Check sheet for the modelled part. Datum: model origin and axes. Units: mm. A direction names the side the tool comes from. Round coordinates to 2 decimals unless told otherwise and drop trailing zeros. Write each loop counter-clockwise with the first axis right and the second up, starting at its lowest first coordinate (ties: lowest second). Pieces come first, ordered by that corner, then holes.
from build123d import *

# Parameters (mm, degrees)
SKETCH1_W                = 51
SKETCH1_H                = 53.5
BOSS_EXTRUDE1_DEPTH      = 54.25
SKETCH2_W                = 43
SKETCH2_H                = 43
CUT_EXTRUDE1_DEPTH       = 50.75
SKETCH3_W                = 43
SKETCH3_H                = 3.5
CUT_EXTRUDE2_DEPTH       = 37.5
CUT_EXTRUDE3_DEPTH       = 76
SKETCH5_R                = 9.673114497
SKETCH5_R_2              = 5.390775308
SKETCH5_R_3              = 5.456912487
CUT_EXTRUDE4_DEPTH       = 76
SKETCH6_R                = 14
SKETCH6_R_2              = 1.75
CUT_EXTRUDE5_DEPTH       = 76
SKETCH7_R                = 5
CUT_EXTRUDE6_DEPTH       = 76
CUT_EXTRUDE7_DEPTH       = 27
FILLET2_R                = 1
SKETCH12_R               = 1.75
CUT_EXTRUDE8_DEPTH       = 15
BOSS_EXTRUDE4_DEPTH      = 10
BOSS_EXTRUDE4_DEPTH_BACK = 61
SKETCH13_W               = 16.75
SKETCH13_H               = 3.5
SKETCH14_W               = 71
SKETCH14_H               = 1.75
BOSS_EXTRUDE5_DEPTH      = 15
SKETCH15_R               = 1.75
CUT_EXTRUDE9_DEPTH       = 10
SKETCH16_R               = 1.75
CUT_EXTRUDE10_DEPTH      = 10
CUT_EXTRUDE11_REACH      = 95.245
FILLET3_R                = 5
FILLET4_R                = 1
CUT_EXTRUDE12_DEPTH      = 2.5


with BuildPart() as part:
    # Sketch1 → Boss-Extrude1 (new body)
    with BuildSketch(Plane.XY):
        with Locations((-26.432354029, 2.021717979)):
            Rectangle(SKETCH1_W, SKETCH1_H)
    extrude(amount=BOSS_EXTRUDE1_DEPTH)

    # Sketch2 → Cut-Extrude1 (cut)
    with BuildSketch(Plane.XY.offset(54.25)):
        with Locations((-26.432354029, 3.771717979)):
            Rectangle(SKETCH2_W, SKETCH2_H)
    extrude(amount=-CUT_EXTRUDE1_DEPTH, mode=Mode.SUBTRACT)

    # Sketch3 → Cut-Extrude2 (cut)
    with BuildSketch(Plane.XY.offset(54.25)):
        with Locations((-26.432354029, 27.021717979)):
            Rectangle(SKETCH3_W, SKETCH3_H)
    extrude(amount=-CUT_EXTRUDE2_DEPTH, mode=Mode.SUBTRACT)

    # Sketch4 → Cut-Extrude3 (cut)
    with BuildSketch(Plane.ZY.offset(51.932354029)):
        with BuildLine():
            Line((16.75, 28.771717979), (54.25, 28.771717979))
            Line((54.25, 28.771717979), (54.25, -7.074674815))
            ThreePointArc((54.25, -7.074674815), (27.422353926, 2.398250742), (16.75, 28.771717979))
        make_face()
    extrude(amount=-CUT_EXTRUDE3_DEPTH, mode=Mode.SUBTRACT)

    # Sketch5 → Cut-Extrude4 (cut)
    with BuildSketch(Plane.ZY.offset(51.932354029)):
        with Locations(Location((14.525222974, -6.808047023, 0), (0, 0, 270))):
            Circle(SKETCH5_R)
        with Locations(Location((34.168969833, -12.297713654, 0), (0, 0, 270))):
            Circle(SKETCH5_R_2)
        with Locations(Location((9.035556344, 13.166402645, 0), (0, 0, 270))):
            Circle(SKETCH5_R_3)
    extrude(amount=-CUT_EXTRUDE4_DEPTH, mode=Mode.SUBTRACT)

    # Sketch6 → Cut-Extrude5 (cut)
    with BuildSketch(Plane.XY.offset(3.5)):
        with Locations((-26.432354029, 3.771717979)):
            Circle(SKETCH6_R)
        with Locations((-10.932354029, 19.271717979)):
            Circle(SKETCH6_R_2)
        with Locations((-41.932354029, 19.271717979)):
            Circle(SKETCH6_R_2)
        with Locations((-41.932354029, -11.728282021)):
            Circle(SKETCH6_R_2)
        with Locations((-10.932354029, -11.728282021)):
            Circle(SKETCH6_R_2)
    extrude(amount=-CUT_EXTRUDE5_DEPTH, mode=Mode.SUBTRACT)

    # Sketch7 → Cut-Extrude6 (cut)
    with BuildSketch(Plane(origin=(0, 0, 0), x_dir=(-1, 0, 0), z_dir=(0, 0, -1))):
        with Locations((26.432354029, -24.728282021)):
            Circle(SKETCH7_R)
    extrude(amount=-CUT_EXTRUDE6_DEPTH, mode=Mode.SUBTRACT)

    # Sketch8 → Cut-Extrude7 (cut)
    with BuildSketch(Plane.XZ.offset(24.728282021)):
        Polygon((-26.432354029, 46.625), (-6.932354029, 27.125), (-26.432354029, 7.625), (-45.932354029, 27.125), align=None)
        Polygon((-13.361286217, 40.625), (-4.932354029, 40.625), (-4.932354029, 32.196067812), align=None)
        Polygon((-4.932354029, 13.625), (-13.361286217, 13.625), (-4.932354029, 22.053932188), align=None)
        Polygon((-47.932354029, 13.625), (-39.503421841, 13.625), (-47.932354029, 22.053932188), align=None)
        Polygon((-47.932354029, 40.625), (-39.007101497, 40.625), (-47.932354029, 31.699747468), align=None)
    extrude(amount=-CUT_EXTRUDE7_DEPTH, mode=Mode.SUBTRACT)

    # Fillet2
    fillet2_edges = [part.edges().sort_by_distance(p)[0] for p in [
        (-47.932354029, -21.228282021, 31.699747468),
        (-4.932354029, -21.228282021, 32.196067812),
        (-4.932354029, -21.228282021, 22.053932188),
        (-47.932354029, -21.228282021, 22.053932188),
        (-13.361286217, -21.228282021, 13.625),
        (-39.503421841, -21.228282021, 13.625),
        (-26.432354029, -18.728282021, 7.625),
        (-4.932354029, -21.228282021, 13.625),
        (-47.932354029, -21.228282021, 13.625),
        (-45.932354029, -21.228282021, 27.125),
        (-6.932354029, -21.228282021, 27.125),
        (-4.932354029, -21.228282021, 40.625),
        (-47.932354029, -21.228282021, 40.625),
        (-39.007101497, -21.228282021, 40.625),
        (-13.361286217, -21.228282021, 40.625),
        (-26.432354029, -18.728282021, 46.625),
    ]]
    fillet(fillet2_edges, radius=FILLET2_R)

    # Sketch12 → Cut-Extrude8 (cut)
    with BuildSketch(Plane.XZ.offset(24.728282021)):
        with Locations(Location((-11.432354029, 46.25, 0), (0, 0, 270))):
            Circle(SKETCH12_R)
        with Locations(Location((-41.432354029, 46.25, 0), (0, 0, 270))):
            Circle(SKETCH12_R)
        with Locations(Location((-11.432354029, 8, 0), (0, 0, 270))):
            Circle(SKETCH12_R)
        with Locations(Location((-41.432354029, 8, 0), (0, 0, 270))):
            Circle(SKETCH12_R)
    extrude(amount=-CUT_EXTRUDE8_DEPTH, mode=Mode.SUBTRACT)

    # Sketch13 → Boss-Extrude4 (add, two sides: drawn at the far end of the back side and taken through both)
    with BuildSketch(Plane.ZY.offset(51.932354029).offset(-BOSS_EXTRUDE4_DEPTH_BACK)):
        with Locations((8.375, 27.021717979)):
            Rectangle(SKETCH13_W, SKETCH13_H)
    extrude(amount=BOSS_EXTRUDE4_DEPTH + BOSS_EXTRUDE4_DEPTH_BACK)

    # Sketch14 → Boss-Extrude5 (add)
    with BuildSketch(Plane(origin=(0, 28.771717979, 0), x_dir=(1, 0, 0), z_dir=(0, 1, 0))):
        with Locations((-26.432354029, -0.875)):
            Rectangle(SKETCH14_W, SKETCH14_H)
    extrude(amount=BOSS_EXTRUDE5_DEPTH)

    # Sketch15 → Cut-Extrude9 (cut)
    with BuildSketch(Plane.XZ.offset(-25.271717979)):
        with Locations((-56.932354029, 9.25)):
            Circle(SKETCH15_R)
        with Locations((4.067645971, 9.25)):
            Circle(SKETCH15_R)
    extrude(amount=-CUT_EXTRUDE9_DEPTH, mode=Mode.SUBTRACT)

    # Sketch16 → Cut-Extrude10 (cut)
    with BuildSketch(Plane(origin=(0, 0, 0), x_dir=(-1, 0, 0), z_dir=(0, 0, -1))):
        with Locations((54.432354029, 36.271717979)):
            Circle(SKETCH16_R)
        with Locations((-1.567645971, 36.271717979)):
            Circle(SKETCH16_R)
        with Locations((44.432354029, 36.271717979)):
            Circle(SKETCH16_R)
        with Locations((8.432354029, 36.271717979)):
            Circle(SKETCH16_R)
    extrude(amount=-CUT_EXTRUDE10_DEPTH, mode=Mode.SUBTRACT)

    # Cut-Extrude11: up to this face of the body (flat: up to its plane)
    cut_extrude11_end = Plane(part.part.faces().sort_by_distance((-26.432354029, -17.120170189, 3.5))[0])
    # Sketch17 → Cut-Extrude11 (cut, up to the picked face)
    with BuildSketch(Plane.XY.offset(54.25), mode=Mode.PRIVATE) as cut_extrude11_sk1:
        with BuildLine():
            Line((-17.488082119, -19.228282021), (-4.932354029, -19.228282021))
            Line((-4.932354029, -19.228282021), (-4.932354029, -17.728282021))
            Line((-4.932354029, -17.728282021), (-18.606116108, -17.728282021))
            ThreePointArc((-18.606116108, -17.728282021), (-18.013624909, -18.453331822), (-17.488082119, -19.228282021))
        make_face()
    cut_extrude11_tool1 = split(extrude(cut_extrude11_sk1.sketch, amount=-CUT_EXTRUDE11_REACH, mode=Mode.PRIVATE), bisect_by=cut_extrude11_end, keep=Keep.BOTH, mode=Mode.PRIVATE)
    # Sketch17 → Cut-Extrude11 (cut, up to the picked face)
    with BuildSketch(Plane.XY.offset(54.25), mode=Mode.PRIVATE) as cut_extrude11_sk2:
        with BuildLine():
            Line((-35.376625939, -19.228282021), (-47.932354029, -19.228282021))
            Line((-47.932354029, -19.228282021), (-47.932354029, -17.728282021))
            Line((-47.932354029, -17.728282021), (-34.25859195, -17.728282021))
            ThreePointArc((-34.25859195, -17.728282021), (-34.851083149, -18.453331822), (-35.376625939, -19.228282021))
        make_face()
    cut_extrude11_tool2 = split(extrude(cut_extrude11_sk2.sketch, amount=-CUT_EXTRUDE11_REACH, mode=Mode.PRIVATE), bisect_by=cut_extrude11_end, keep=Keep.BOTH, mode=Mode.PRIVATE)
    add(cut_extrude11_tool1.solids().sort_by(Axis((-11.476334, -18.467624, 54.25), (0, 0, -1)))[0], mode=Mode.SUBTRACT)
    add(cut_extrude11_tool2.solids().sort_by(Axis((-41.388374, -18.467624, 54.25), (0, 0, -1)))[0], mode=Mode.SUBTRACT)

    # Fillet3
    fillet3_edges = [part.edges().sort_by_distance(p)[0] for p in [
        (-2.932354029, -7.074674815, 54.25),
        (-49.932354029, -7.074674815, 54.25),
    ]]
    fillet(fillet3_edges, radius=FILLET3_R)

    # Fillet4
    fillet4_edges = [part.edges().sort_by_distance(p)[0] for p in [
        (-51.932354029, 25.271717979, 8.375),
        (-0.932354029, 25.271717979, 8.375),
        (-0.932354029, -24.728282021, 27.125),
        (-51.932354029, -24.728282021, 27.125),
    ]]
    fillet(fillet4_edges, radius=FILLET4_R)

    # Sketch19 → Cut-Extrude12 (cut)
    with BuildSketch(Plane(origin=(0, -19.228282021, 0), x_dir=(1, 0, 0), z_dir=(0, 1, 0))):
        Polygon((-44.182354029, -9.58771324), (-41.432354029, -11.175426481), (-38.682354029, -9.58771324), (-38.682354029, -6.41228676), (-41.432354029, -4.824573519), (-44.182354029, -6.41228676), align=None)
        Polygon((-11.432354029, -4.824573519), (-14.182354029, -6.41228676), (-14.182354029, -9.58771324), (-11.432354029, -11.175426481), (-8.682354029, -9.58771324), (-8.682354029, -6.41228676), align=None)
        Polygon((-38.682354029, -47.83771324), (-38.682354029, -44.66228676), (-41.432354029, -43.074573519), (-44.182354029, -44.66228676), (-44.182354029, -47.83771324), (-41.432354029, -49.425426481), align=None)
        Polygon((-8.682354029, -47.83771324), (-8.682354029, -44.66228676), (-11.432354029, -43.074573519), (-14.182354029, -44.66228676), (-14.182354029, -47.83771324), (-11.432354029, -49.425426481), align=None)
    extrude(amount=-CUT_EXTRUDE12_DEPTH, mode=Mode.SUBTRACT)


solid = part.part
1. Release check for a two-part mould opening along Z. For faces 1 (the flat face through (-42.83, -20.46, 48.62)), 2 (the flat face through (6, 25.272, 8)), 3 (the flat face through (-36, -7, 3.5)), 4 (the flat face through (-8.682, -20, 8)) record: released by +Z, released by -Z, zero draft, split by the parting line, or undercut.
2. Sectioned sample at B-B, the plane y = 12.5. Enter the section's corners in (x, z).
3. Scan lines: line 1 along Z through (x, y) = (-1, 13.5); line 2 along X through (y, z) = (9, 5); line 3 along Y through (x, z) = (-44, 9.5). Record each from-to range of solid material in increasing order.
4. Go/stop test with flat-tipped pins: pin 1 (3 mm diameter, centred on x = -51.5, z = 28, fed in from -Y); pin 2 (3 mm diameter, centred on x = -41.43, z = 8, fed in from -Y); pin 3 (3 mm diameter, centred on x = -18.5, y = 18, fed in from +Z); pin 4 (6 mm diameter, centred on x = -10.5, z = 47, fed in from +Y). Record where each tip stops, or that it passes through.
5. Sectioned sample at D-D, the plane z = 32. Enter the section's corners in (x, y), plus the area to 3 significant figures.
6. Sectioned sample at C-C, the plane x = -20.5. Enter the section's corners in (y, z), plus the area to 3 significant figures.
7. Sectioned sample at A-A, the plane z = 23. Enter the section's corners in (x, y), plus the area to 3 significant figures.
8. Set-up check for faces 5 (the flat face through (-27, 25.272, 10)), 6 (the flat face through (-40.04, -20.46, 5.63)), 7 (the flat face through (-51.932, -5, 27)), 8 (the flat face through (-16.56, -21.28, 17.5)), 9 (the cylindrical face through (-40.504, -21.94, 40.023)): record each of +Z, -Z, +X, -X, +Y, -Y from which the full face is reachable in a straight line by a thin tool's end or side.
Computed values:
1. face 1: undercut
1. face 2: zero draft
1. face 3: released by +Z
1. face 4: undercut
2. outline: (-51.93, 0) - (-37.38, 0) - (-37.38, 3.5) - (-47.93, 3.5) - (-47.93, 3.62) - (-51.93, 3.62) - close; (-51.93, 14.45) - (-47.93, 14.45) - (-47.93, 20.11) - (-51.93, 20.11) - close; (-15.49, 0) - (-0.93, 0) - (-0.93, 3.62) - (-4.93, 3.62) - (-4.93, 3.5) - (-15.49, 3.5) - close; (-4.93, 14.45) - (-0.93, 14.45) - (-0.93, 20.11) - (-4.93, 20.11) - close
3. line 1: z = 0 to 3.59, 14.48 to 19.65
3. line 2: x = -51.93 to -47.93, -4.93 to -0.93
3. line 3: y = -24.73 to -21.73, 25.27 to 28.77
4. pin 1: stops at y = -24.73
4. pin 2: stops at y = 25.27
4. pin 3: stops at z = 3.5
4. pin 4: stops at y = -19.23
5. outline: (-51.93, -23.73) arc R1 ccw to (-50.93, -24.73) - (-41.06, -24.73) - (-41.06, -19.23) - (-47.93, -19.23) - (-47.93, -17.23) - (-51.93, -17.23) - close; (-51.93, -7.36) - (-47.93, -7.36) - (-47.93, -1.29) - (-51.93, -1.29) - close; (-11.81, -24.73) - (-1.93, -24.73) arc R1 ccw to (-0.93, -23.73) - (-0.93, -17.23) - (-4.93, -17.23) - (-4.93, -19.23) - (-11.81, -19.23) - close; (-4.93, -7.36) - (-0.93, -7.36) - (-0.93, -1.29) - (-4.93, -1.29) - close
5. area: 184 mm2
6. outline: (-24.73, 0) - (-8.91, 0) - (-8.91, 3.5) - (-17.73, 3.5) - (-17.73, 13.56) - (-24.73, 13.56) - close; (-24.73, 40.69) - (-17.73, 40.69) - (-17.73, 54.25) - (-24.73, 54.25) - close; (16.45, 0) - (43.77, 0) - (43.77, 1.75) - (28.77, 1.75) - (28.77, 16.75) - (25.27, 16.75) - (25.27, 3.5) - (16.45, 3.5) - close
6. area: 336 mm2
7. outline: (-51.93, -23.73) arc R1 ccw to (-50.93, -24.73) - (-41.81, -24.73) - (-41.81, -19.23) - (-47.93, -19.23) - (-47.93, -11.47) - (-51.93, -11.47) - close; (-51.93, -2.14) - (-47.93, -2.14) - (-47.93, 7.55) - (-51.93, 7.55) - close; (-11.06, -24.73) - (-1.93, -24.73) arc R1 ccw to (-0.93, -23.73) - (-0.93, -11.47) - (-4.93, -11.47) - (-4.93, -19.23) - (-11.06, -19.23) - close; (-4.93, -2.14) - (-0.93, -2.14) - (-0.93, 7.55) - (-4.93, 7.55) - close
7. area: 251 mm2
8. face 5: +Z
8. face 6: none
8. face 7: +Z, -Z, -X, -Y
8. face 8: -Y
8. face 9: +Y, -Y
